Could you check a few things on this model? Use its own coordinates, in mm. A direction names the side the tool comes from. Round coordinates to 2 decimals unless told otherwise and drop trailing zeros. Write each loop counter-clockwise with the first axis right and the second up, starting at its lowest first coordinate (ties: lowest second). Pieces come first, ordered by that corner, then holes. Notation, with made-up numbers: (73.25, 73) - (92.25, 73) arc R25 ccw to (92.25, 99) - close; hole circle Ø3 at (39.25, 78). An arc over 180 degrees is marked (long way). Write each question's results on one line, items separated by ' | '. Start each with the question number.
(1) For P1, Ø3, axis at x = 2, z = -63.5, coming from the -Y side; P2, Ø12, axis at x = 44.5, y = 3, coming from the +Z side; P3, Ø1, axis at y = -10, z = -34, coming from the +X side, each with a flat end and sliding along its axis, tell me the tip position at first contact or that it passes through.
(2) Thinking about a two-plate mould opening in Z: for faces 4 (the flat face through (75.5, -6, -53)), 5 (the flat face through (77.5, -3, -54)), 6 (the cylindrical face through (0.1, 86, -57.9)), which applies, +Z half, -Z half, draft (parallel to the pull), parting line (faces both ways), or undercut?
(3) Imagine slicing it at C-C on x = -27. Write out the boundary of the cut face in (y, z), then the cut area to 3 significant figures.
(4) Please list where these lines run through material, in increasing order: line 1 (X direction, y = -48.5, z = -64); line 2 (X direction, y = 86, z = -62); line 3 (Y direction, x = -15.5, z = -63.5). Write a range as [from, to].
(5) On a 3-axis mill with a long thin cutter (end or side, diameter ignored), from which of +Z, -Z, +X, -X, +Y, -Y can I reach the whole of each face in a straight line? I mean faces 1 (the flat face through (-0.1, 84.5, -67.3)), 2 (the flat face through (74.486, -5.281, -37.709)), 3 (the flat face through (0, -97.5, -72)). Say none if no direction works.
(6) Imagine slicing it at D-D on y = 30. Write out the boundary of the cut face in (x, z), then the cut area to 3 significant figures.
(7) Imagine slicing it at B-B on y = -82. Write out the boundary of the cut face in (x, z), then the cut area to 3 significant figures.
(8) Imagine slicing it at A-A on z = -51.5. Write out the boundary of the cut face in (x, y).
```python
from build123d import *

# Parameters (mm, degrees)
SKETCH049_W  = 155
SKETCH049_H  = 187
PAD013_DEPTH = 2
PAD014_DEPTH = 36
PAD015_DEPTH = 183
SKETCH055_W  = 1.8
SKETCH055_H  = 129.8
PAD016_DEPTH = 2
SKETCH081_R  = 4.05
PAD027_DEPTH = 3


with BuildPart() as part:
    # Sketch049 → Pad013 (new body)
    with BuildSketch(Plane.XY):
        with Locations((0, -4)):
            Rectangle(SKETCH049_W, SKETCH049_H)
    extrude(amount=PAD013_DEPTH)

    # Sketch050 (on DatumPlane) → Pad014 (join)
    with BuildSketch(Plane.XY.offset(2)):
        Polygon((-77.5, -97.5), (-77.5, 89.5), (77.5, 89.5), (77.5, -97.5), (75.5, -97.5), (75.5, 87.5), (-75.5, 87.5), (-75.5, -97.5), align=None)
    extrude(amount=PAD014_DEPTH)

    # Sketch051 (on DatumPlane) → Pad015 (join)
    with BuildSketch(Plane.XZ.offset(95.5)):
        Polygon((-75.5, 32.505045), (-75.5, 38), (-73.5, 38), align=None)
    pad015 = extrude(amount=-PAD015_DEPTH)

    # Mirrored006: Pad015 across Sketch051 V_Axis
    add(pad015.mirror(Plane(origin=(0, -95.5, 0), x_dir=(0, -1, 0), z_dir=(1, 0, 0))))

    # Sketch055 (on DatumPlane) → Pad016 (join)
    with BuildSketch(Plane.XY.offset(38)):
        with Locations((74.5, 0)):
            Rectangle(SKETCH055_W, SKETCH055_H)
    pad016 = extrude(amount=PAD016_DEPTH)

    # Mirrored008: Pad016 across Sketch055 V_Axis
    add(pad016.mirror(Plane(origin=(0, 0, 38), x_dir=(0, 0, 1), z_dir=(1, 0, 0))))

    # Sketch081 (on DatumPlane) → Pad027 (join)
    with BuildSketch(Plane.XZ.offset(-87.5)):
        with BuildLine():
            ThreePointArc((5.05, 10.05), (0, 15.1), (-5.05, 10.05))
            Line((-5.05, 10.05), (-5.05, 2))
            Line((-5.05, 2), (5.05, 2))
            Line((5.05, 2), (5.05, 10.05))
        make_face()
        with Locations((0, 10.05)):
            Circle(SKETCH081_R, mode=Mode.SUBTRACT)
    extrude(amount=PAD027_DEPTH)


with BuildPart() as part_1:
    # Body006 placement: moved
    add(part.part.moved(Location((0, 0, -73))))


solid = part_1.part
```
Response:
1) P1: y = 87.5 | P2: z = -71 | P3: x = 75.4
2) face 4: undercut | face 5: draft | face 6: +Z half
3) outline: (-97.5, -73) - (89.5, -73) - (89.5, -35) - (87.5, -35) - (87.5, -71) - (-97.5, -71) - close | area: 446 mm²
4) line 1: [-77.5, -75.5], [75.5, 77.5] | line 2: [-77.5, -75.5], [-4.96, -3.94], [3.94, 4.96], [75.5, 77.5] | line 3: [87.5, 89.5]
5) face 1: +Z, -Y | face 2: -Y | face 3: +Z, -Z, +X, -X, -Y
6) outline: (-77.5, -73) - (77.5, -73) - (77.5, -35) - (75.4, -35) - (75.4, -33) - (73.6, -33) - (73.6, -35) - (73.5, -35) - (75.5, -40.49) - (75.5, -71) - (-75.5, -71) - (-75.5, -40.49) - (-73.5, -35) - (-73.6, -35) - (-73.6, -33) - (-75.4, -33) - (-75.4, -35) - (-77.5, -35) - close | area: 472 mm²
7) outline: (-77.5, -73) - (77.5, -73) - (77.5, -35) - (73.5, -35) - (75.5, -40.49) - (75.5, -71) - (-75.5, -71) - (-75.5, -40.49) - (-73.5, -35) - (-77.5, -35) - close | area: 465 mm²
8) outline: (-77.5, -97.5) - (-75.5, -97.5) - (-75.5, 87.5) - (75.5, 87.5) - (75.5, -97.5) - (77.5, -97.5) - (77.5, 89.5) - (-77.5, 89.5) - close
